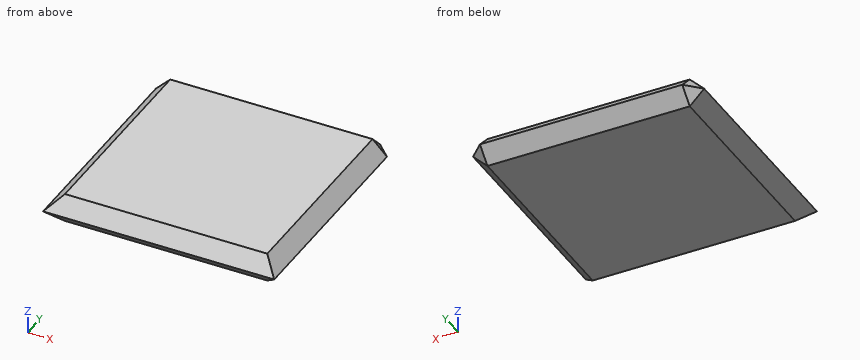
from build123d import *

# Parameters (mm, degrees)
F0_W     = 80
F0_H     = 80
F1_DEPTH = 10
F2_SIZE  = 4.99999


# Not quite as in the source:
# - a fillet or chamfer is up to 0.001 mm smaller than in the source, because OpenCascade refuses the exact size


with BuildPart() as f1:
    # F0 (on Top) → F1 (new body)
    with BuildSketch(Plane.XY):
        with Locations((40, -40)):
            Rectangle(F0_W, F0_H)
    extrude(amount=F1_DEPTH)

    # F2 (size 5 in the source; OpenCascade refuses exactly that, so slightly less here)
    f2_edges = [f1.edges().sort_by_distance(p)[0] for p in [
        (40, 0, 0),
        (40, 0, 10),
        (0, 0, 5),
        (80, 0, 5),
        (80, -40, 0),
        (80, -40, 10),
        (40, -80, 0),
        (40, -80, 10),
        (0, -40, 0),
        (0, -40, 10),
    ]]
    chamfer(f2_edges, length=F2_SIZE)


solid = f1.part
Input: part model. Units: mm. Frame: model coordinates. Give positions to 0.01 mm unless a question says otherwise; leave off trailing zeros. Loops run counter-clockwise (first coordinate to the right, second up) from the corner with the lowest first, then second, coordinate; pieces in that order, holes last. Notation, with made-up numbers: (-10, -21.75) - (-1, -21.75) arc R25 ccw to (-1, 8.25) - close; hole circle Ø6 at (57, 84.5). An arc over 180 degrees is marked (long way). Use CSV: the item, a comma, the result in double quotes. Start each with the question number.
Item 1: Line query: line 1 (Y direction, x = 74.5, z = 2.25); line 2 (X direction, y = -17.5, z = 9); line 3 (Y direction, x = 52, z = 7). Output: solid intervals per line, ascending.
Item 2: Section C-C on z = 3. Return loops of the section in (x, y), then the cut area to 3 significant figures.
Item 3: Contact query for flat-ended pins moving along their axis: P1, Ø3, axis at y = -52, z = 7.5, coming from the +X side; P2, Ø1.5, axis at y = -55.5, z = 8, coming from the +X side; P3, Ø3, axis at x = 53, z = 4, coming from the +Y side. Output: stop coordinate, or through.
Item 4: Section D-D on z = 8.25. Return loops of the section in (x, y).
Ans:
1,line 1,"y = -77.25 to -2.75"
1,line 2,"x = 4 to 76"
1,line 3,"y = -78 to -2"
2,outline,"(2, -78) - (78, -78) - (78, -5) - (75, -2) - (5, -2) - (2, -5) - close"
2,area,"5,770 mm2"
3,P1,"stops at x = 79"
3,P2,"stops at x = 77.75"
3,P3,"stops at y = 0"
4,outline,"(3.25, -76.75) - (76.75, -76.75) - (76.75, -5) - (75, -3.25) - (5, -3.25) - (3.25, -5) - close"
